```python
from build123d import *

# Parameters (mm, degrees)
F0_W     = 47.1180379391
F0_H     = 20.1085954905
F1_DEPTH = 6.35
F2_D     = 6.35
F2_DEPTH = 6.351
F4_D     = 6.35


with BuildPart() as f1:
    # F0 (on Front) → F1 (new body, symmetric)
    with BuildSketch(Plane.XZ):
        Rectangle(F0_W, F0_H)
    extrude(amount=F1_DEPTH, both=True)

    # F2 (through all, one way)
    with BuildSketch(Plane(origin=(0, 0, 0), x_dir=(1, 0, 0), z_dir=(0, 1, 0))):
        with Locations((-12.2772194445, 0)):
            Circle(F2_D / 2)
    extrude(amount=-F2_DEPTH, mode=Mode.SUBTRACT)

    # F4 (through all)
    with Locations(Plane.XZ.offset(6.35)):
        with Locations((10.6193870306, 0)):
            Hole(F4_D / 2)


solid = f1.part
```
Here's how the part is built. I have some questions about the finished solid (model axes, mm). A direction names the side the tool comes from. Coordinates: 2 decimals unless noted, no trailing zeros. Order: outer loops, then holes, each group sorted by start corner. A loop starts at its lowest first (then second) coordinate and runs counter-clockwise, first axis right, second up. Notation, with made-up numbers: M -36.5,77.25 L -0.5,77.25 A32 cw -0.5,104.25 Z; hole C 29,78 d3. An arc over 180 degrees is marked long. Answer as a JSON object with one key per item and string values. Group by question number.
(1) Suppose I cut it at D-D, the plane y = -2.5. Please give me the cut outline in (x, z) (3 decimals), then the cut area to 3 significant figures.
(2) Suppose I cut it at A-A, the plane z = 0. Please give me the cut outline in (x, y).
(3) If we mould it in two halves opening along Z, with no side actions, what happens to faces 3 (the face through (-9.249, -3.131, -0.954)), 4 (the face through (23.559, 0, 0)), 5 (the face through (0, 0, 10.054)), 6 (the face through (0, 0, -10.054))? For each: released by +Z, released by -Z, zero draft, split by the parting line, or undercut.
(4) Which directions (+Z, -Z, +X, -X, +Y, -Y) give clear straight access to the entire face, cutting with the end or side of a thin tool? Please do faces 1 (the face through (7.59, 0.09, 0.95)), 2 (the face through (-12, 0, 0)).
(5) For pin 1 (10 mm diameter, centred on x = 10.62, z = 0, fed in from -Y); pin 2 (5.5 mm diameter, centred on x = -12.28, z = 0, fed in from -Y), each with a flat end and sliding along its axis, tell me the tip position at first contact or that it passes through.
(6) I need wall thicknesses on probe 1 along Y at (x, z) = (-15, -1.5); probe 2 along Z at (x, y) = (-14.5, -4.5). Which ranges of each line are inside material? Lowest first, please.
(7) Suppose I cut it at C-C, the plane x = 13. Please give me the cut outline in (y, z), then the cut area to 3 significant figures.
(8) Suppose I cut it at B-B, the plane y = 4.25. Please give me the cut outline in (x, z) (3 decimals).
Values found:
{
 "1": {"outline": "M -23.559,-10.054 L 23.559,-10.054 L 23.559,10.054 L -23.559,10.054 Z; hole C -12.277,0 d6.35; hole C 10.619,0 d6.35", "area": "884 mm^2"},
 "2": {"outline": "M -23.56,-6.35 L -15.45,-6.35 L -15.45,0 L -9.1,0 L -9.1,-6.35 L 7.44,-6.35 L 7.44,6.35 L -23.56,6.35 Z; M 13.79,-6.35 L 23.56,-6.35 L 23.56,6.35 L 13.79,6.35 Z"},
 "3": {"face 3": "undercut", "face 4": "zero draft", "face 5": "released by +Z", "face 6": "released by -Z"},
 "4": {"face 1": "+Y, -Y", "face 2": "-Y"},
 "5": {"pin 1": "stops at y = -6.35", "pin 2": "stops at y = 0"},
 "6": {"probe 1": "y = 0 to 6.35", "probe 2": "z = -10.05 to -2.27, 2.27 to 10.05"},
 "7": {"outline": "M -6.35,-10.05 L 6.35,-10.05 L 6.35,-2.1 L -6.35,-2.1 Z; M -6.35,2.1 L 6.35,2.1 L 6.35,10.05 L -6.35,10.05 Z", "area": "202 mm^2"},
 "8": {"outline": "M -23.559,-10.054 L 23.559,-10.054 L 23.559,10.054 L -23.559,10.054 Z; hole C 10.619,0 d6.35"}
}
